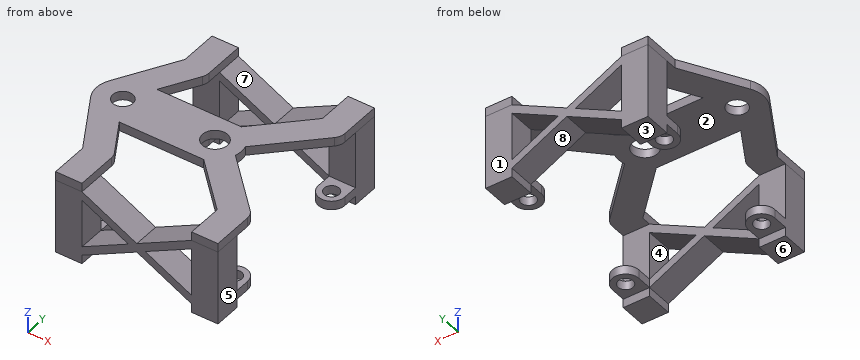
from build123d import *

# Parameters (mm, degrees)
SKETCH094_R                     = 2.3
SKETCH094_R_2                   = 2.85
PAD048_DEPTH                    = 2
SKETCH097_W                     = 6
SKETCH097_H                     = 6
PAD050_DEPTH                    = 17
SKETCH098_R                     = 1.7
PAD051_DEPTH                    = 2
SKETCH098_LINEARPATTERN001_2_R  = 1.7
PAD051_LINEARPATTERN001_2_DEPTH = 2
SKETCH097_LINEARPATTERN001_2_W  = 6
SKETCH097_LINEARPATTERN001_2_H  = 6
PAD050_LINEARPATTERN001_2_DEPTH = 17
PAD052_DEPTH                    = 6


with BuildPart() as part:
    # Sketch094 → Pad048 (new body)
    with BuildSketch(Plane.XY):
        with BuildLine():
            Line((3.464102, 6), (21, 6))
            Line((22.716302, 6), (21, 6))
            Line((22.716302, 6), (33.500258, 16.783955))
            Line((33.500258, 16.783955), (33.500258, 24.930573))
            Line((33.500258, 24.930573), (39.500258, 24.930573))
            Line((39.500258, 24.930573), (39.500258, 15.5))
            ThreePointArc((38.650792, 13.449208), (39.279489, 14.390119), (39.500258, 15.5))
            Line((26.786802, 1.585219), (38.650792, 13.449208))
            ThreePointArc((26.786802, -1.585219), (27, 0), (26.786802, 1.585219))
            Line((26.786802, -1.585219), (38.650792, -13.449208))
            ThreePointArc((39.500258, -15.5), (39.279489, -14.390119), (38.650792, -13.449208))
            Line((39.500258, -24.930573), (39.500258, -15.5))
            Line((33.500258, -24.930573), (39.500258, -24.930573))
            Line((33.500258, -16.783955), (33.500258, -24.930573))
            Line((22.716302, -6), (33.500258, -16.783955))
            Line((21, -6), (22.716302, -6))
            Line((3.464102, -6), (21, -6))
            Line((3.464102, -6), (8.111697, -14.049871))
            ThreePointArc((8.500258, -15.5), (8.401434, -14.749358), (8.111697, -14.049871))
            Line((8.500258, -24.930573), (8.500258, -15.5))
            Line((2.500258, -24.930573), (8.500258, -24.930573))
            Line((2.500258, -16.330573), (2.500258, -24.930573))
            Line((-5.196152, -3), (2.500258, -16.330573))
            ThreePointArc((-5.196152, 3), (-6, 0), (-5.196152, -3))
            Line((-5.196152, 3), (2.500258, 16.330573))
            Line((2.500258, 16.330573), (2.500258, 24.930573))
            Line((2.500258, 24.930573), (8.500258, 24.930573))
            Line((8.500258, 24.930573), (8.500258, 15.5))
            ThreePointArc((8.111697, 14.049871), (8.401434, 14.749358), (8.500258, 15.5))
            Line((3.464102, 6), (8.111697, 14.049871))
        make_face()
        Circle(SKETCH094_R, mode=Mode.SUBTRACT)
        with Locations((21, 0)):
            Circle(SKETCH094_R_2, mode=Mode.SUBTRACT)
    extrude(amount=PAD048_DEPTH)

    # Sketch097 (on Face33 of Pad048) → Pad050 (join)
    with BuildSketch(Plane(origin=(0, 0, 0), x_dir=(1, 0, 0), z_dir=(0, 0, -1))):
        with Locations((5.5, 21.93)):
            Rectangle(SKETCH097_W, SKETCH097_H)
    pad050 = extrude(amount=PAD050_DEPTH)

    # Sketch098 → Pad051 (join)
    with BuildSketch(Plane.XY.offset(-15)):
        with BuildLine():
            Line((2.5, -18.93), (2.5, -15.5))
            ThreePointArc((8.5, -15.5), (5.5, -12.5), (2.5, -15.5))
            Line((8.5, -18.93), (8.5, -15.5))
            Line((2.5, -18.93), (8.5, -18.93))
        make_face()
        with Locations((5.5, -15.5)):
            Circle(SKETCH098_R, mode=Mode.SUBTRACT)
    pad051 = extrude(amount=PAD051_DEPTH)

    # Sketch098 LinearPattern001 2 → Pad051 LinearPattern001 2 (add)
    with BuildSketch(Plane(origin=(31, 0, -15), x_dir=(1, 0, 0), z_dir=(0, 0, 1))):
        with BuildLine():
            Line((2.5, -18.93), (2.5, -15.5))
            ThreePointArc((8.5, -15.5), (5.5, -12.5), (2.5, -15.5))
            Line((8.5, -18.93), (8.5, -15.5))
            Line((2.5, -18.93), (8.5, -18.93))
        make_face()
        with Locations((5.5, -15.5)):
            Circle(SKETCH098_LINEARPATTERN001_2_R, mode=Mode.SUBTRACT)
    pad051_linearpattern001_2 = extrude(amount=PAD051_LINEARPATTERN001_2_DEPTH)

    # Sketch097 LinearPattern001 2 → Pad050 LinearPattern001 2 (add)
    with BuildSketch(Plane(origin=(31, 0, 0), x_dir=(1, 0, 0), z_dir=(0, 0, -1))):
        with Locations((5.5, 21.93)):
            Rectangle(SKETCH097_LINEARPATTERN001_2_W, SKETCH097_LINEARPATTERN001_2_H)
    pad050_linearpattern001_2 = extrude(amount=PAD050_LINEARPATTERN001_2_DEPTH)

    # Mirrored001: Pad051, Pad050, Pad051 LinearPattern001 2, Pad050 LinearPattern001 2 across Sketch098 H_Axis
    add(pad051.mirror(Plane(origin=(0, 0, -15), x_dir=(0, 0, 1), z_dir=(0, 1, 0))))
    add(pad050.mirror(Plane(origin=(0, 0, -15), x_dir=(0, 0, 1), z_dir=(0, 1, 0))))
    add(pad051_linearpattern001_2.mirror(Plane(origin=(0, 0, -15), x_dir=(0, 0, 1), z_dir=(0, 1, 0))))
    add(pad050_linearpattern001_2.mirror(Plane(origin=(0, 0, -15), x_dir=(0, 0, 1), z_dir=(0, 1, 0))))

    # Sketch099 (on Face36 of MultiTransform001) → Pad052 (join)
    with BuildSketch(Plane.XZ.offset(24.93)):
        Polygon((8.5, 0), (21, -6.5), (33.5, 0), (33.5, -2), (22.923077, -7.5), (33.5, -13), (33.5, -15), (21, -8.5), (8.5, -15), (8.5, -13), (19.076923, -7.5), (8.5, -2), align=None)
    pad052 = extrude(amount=-PAD052_DEPTH)

    # Mirrored002: Pad052 across XZ
    add(pad052.mirror(Plane.XZ))


with BuildPart() as part_1:
    # Body024 placement: moved
    add(part.part.moved(Location((46.5, 0, 31))))


solid = part_1.part
Model file for the job. Use its own axes, mm. Face numbers are marked on the shaded views. A direction names the side the tool comes from. Give positions to 0.01 mm unless a question says otherwise; leave off trailing zeros. Loops run counter-clockwise (first coordinate to the right, second up) from the corner with the lowest first, then second, coordinate; pieces in that order, holes last. Notation, with made-up numbers: (-32, -10.75) -> (25, -10.75) arc R21 cw to (25, -4.75) -> close; hole circle Ø9 at (-27.75, 58). An arc over 180 degrees is marked (long way). Use a Markdown table: item, result. Add a question column.
(1) Slice it at A-A on x = 46.5. List the corners of the cut face in (y, z), and give its area (3 significant figures).
(2) Slice it at C-C on z = 20.75. Give the number of separate pieces and of enclosed holes in the cut face, and give its area (3 significant figures).
(3) Slice it at D-D on x = 76. List the corners of the cut face in (y, z).
(4) Wall check: line 1 along X through (y, z) = (15.5, 17.65); line 2 along Y through (x, z) = (52, 16.45); line 3 along Y through (x, z) = (59, 27). Give the ranges that are in metal, low to high.
(5) Slice it at B-B on y = 0. List the corners of the cut face in (x, z).
(6) Tool access for the marked faces 4, 5, 6, 7 and 8: list every direction of +Z, -Z, +X, -X, +Y, -Y with a clear straight run to the whole face (end or side of a thin tool).
(7) Drop flat-ended pins along their axis: pin 1 Ø9 at (x, y) = (67.5, 0) entering from -Z; pin 2 Ø6.5 at (x, y) = (83.5, 15.5) entering from -Z; pin 3 Ø2 at (y, z) = (22.5, 15) entering from -X. Give the stop position or say it passes through.
(8) Mould opens along Y. For the marked faces 1, 2 and 3 say: +Y half, -Y half, draft (parallel to the pull), parting line (faces both ways), or undercut.
Filled sheet:
| question | item | result |
|---|---|---|
| 1 | outline | (-12, 31) -> (-2.3, 31) -> (-2.3, 33) -> (-12, 33) -> close; (2.3, 31) -> (12, 31) -> (12, 33) -> (2.3, 33) -> close |
| 1 | area | 38.8 mm2 |
| 2 | separate pieces | 8 |
| 2 | enclosed holes | 0 |
| 2 | area | 236 mm2 |
| 3 | outline | (-24.93, 18.08) -> (-18.93, 18.08) -> (-18.93, 20.08) -> (-24.93, 20.08) -> close; (-24.93, 26.92) -> (-18.93, 26.92) -> (-18.93, 28.92) -> (-24.93, 28.92) -> close; (-12.78, 31) -> (-4.3, 31) -> (-4.3, 33) -> (-12.78, 33) -> close; (4.3, 31) -> (12.78, 31) -> (12.78, 33) -> (4.3, 33) -> close; (18.93, 18.08) -> (24.93, 18.08) -> (24.93, 20.08) -> (18.93, 20.08) -> close; (18.93, 26.92) -> (24.93, 26.92) -> (24.93, 28.92) -> (18.93, 28.92) -> close |
| 4 | line 1 | 49 to 50.3, 53.7 to 55, 80 to 81.3, 84.7 to 86 |
| 4 | line 2 | -24.93 to -17.2, -13.8 to -12.5, 12.5 to 13.8, 17.2 to 24.93 |
| 4 | line 3 | -24.93 to -18.93, 18.93 to 24.93 |
| 5 | outline | (40.5, 31) -> (44.2, 31) -> (44.2, 33) -> (40.5, 33) -> close; (48.8, 31) -> (64.65, 31) -> (64.65, 33) -> (48.8, 33) -> close; (70.35, 31) -> (73.5, 31) -> (73.5, 33) -> (70.35, 33) -> close |
| 6 | face 4 | +Y, -Y |
| 6 | face 5 | +Z, -Z, +X, +Y, -Y |
| 6 | face 6 | -Z, +X, -X, +Y, -Y |
| 6 | face 7 | +Z, +Y, -Y |
| 6 | face 8 | -Z, +Y, -Y |
| 7 | pin 1 | z = 31 |
| 7 | pin 2 | z = 16 |
| 7 | pin 3 | x = 49 |
| 8 | face 1 | +Y half |
| 8 | face 2 | undercut |
| 8 | face 3 | draft |
